from build123d import *

# Parameters (mm, degrees)
SKETCH029_W             = 70
SKETCH029_H             = 20
PAD005_DEPTH            = 12.7
SKETCH012_W             = 36
SKETCH012_H             = 17
PAD006_DEPTH            = 40
POCKET016_DEPTH         = 40
POCKET014_DEPTH         = 22.994766
SKETCH027_W             = 36
SKETCH027_H             = 30
PAD007_DEPTH            = 6
POCKET017_DEPTH         = 2
POCKET015_DEPTH         = 22
POCKET015_DEPTH_BACK    = 100
SKETCH013_R             = 9
POCKET018_DEPTH         = 40
FILLET_R                = 1
CHAMFER014_SIZE         = 2
CHAMFER013_SIZE         = 4
BODY002_ROLL_ANGLE      = -123.951696
BODY002_PITCH_ANGLE     = 0.828143
BODY002_PLACEMENT_ANGLE = 179.441913


with BuildPart() as part:
    # Sketch029 → Pad005 (new body)
    with BuildSketch(Plane.XY):
        with Locations((-8, 8)):
            Rectangle(SKETCH029_W, SKETCH029_H)
    extrude(amount=PAD005_DEPTH)

    # Sketch012 (on Face6 of Pad005) → Pad006 (join)
    with BuildSketch(Plane.XY.offset(12.7)):
        with Locations((-8, 9.5)):
            Rectangle(SKETCH012_W, SKETCH012_H)
    extrude(amount=PAD006_DEPTH)

    # Sketch028 → Pocket016 (cut)
    with BuildSketch(Plane.XY.offset(52.7)):
        with BuildLine():
            ThreePointArc((-3, 5), (-8, 10), (-13, 5))
            Line((-13, -7.39), (-13, 5))
            Line((-3, -7.39), (-13, -7.39))
            Line((-3, 5), (-3, -7.39))
        make_face()
    extrude(amount=-POCKET016_DEPTH, mode=Mode.SUBTRACT)

    # Sketch025 → Pocket014 (cut, through all)
    with BuildSketch(Plane(origin=(0, 20.993766, 0), x_dir=(-1, 0, 0), z_dir=(0, 1, 0))):
        with BuildLine():
            ThreePointArc((-16.5, 8.95), (-19.1, 6.35), (-16.5, 3.75))
            Line((-16.5, 3.75), (-14.5, 3.75))
            ThreePointArc((-14.5, 3.75), (-11.9, 6.35), (-14.5, 8.95))
            Line((-16.5, 8.95), (-14.5, 8.95))
        make_face()
        with BuildLine():
            ThreePointArc((30.5, 8.95), (27.9, 6.35), (30.5, 3.75))
            Line((30.5, 3.75), (32.5, 3.75))
            ThreePointArc((32.5, 3.75), (35.1, 6.35), (32.5, 8.95))
            Line((30.5, 8.95), (32.5, 8.95))
        make_face()
    extrude(amount=-POCKET014_DEPTH, mode=Mode.SUBTRACT)

    # Sketch027 → Pad007 (join)
    with BuildSketch(Plane.XY.offset(52.7)):
        with Locations((-8, 3)):
            Rectangle(SKETCH027_W, SKETCH027_H)
        with BuildLine():
            ThreePointArc((-19.25, -7), (-21, -5.25), (-22.75, -7))
            Line((-22.75, -7), (-22.75, -9))
            ThreePointArc((-22.75, -9), (-21, -10.75), (-19.25, -9))
            Line((-19.25, -7), (-19.25, -9))
        make_face(mode=Mode.SUBTRACT)
        with BuildLine():
            ThreePointArc((6.75, -7), (5, -5.25), (3.25, -7))
            Line((3.25, -7), (3.25, -9))
            ThreePointArc((3.25, -9), (5, -10.75), (6.75, -9))
            Line((6.75, -7), (6.75, -9))
        make_face(mode=Mode.SUBTRACT)
    extrude(amount=PAD007_DEPTH)

    # Sketch026 → Pocket017 (cut)
    with BuildSketch(Plane.XY.offset(56.7)):
        Polygon((5.856406, 5), (-1.071797, 17), (-14.928203, 17), (-21.856406, 5), (-14.928203, -7), (-1.071797, -7), align=None)
    extrude(amount=POCKET017_DEPTH, mode=Mode.SUBTRACT)

    # Sketch030 → Pocket015 (cut, two sides)
    with BuildSketch(Plane.XY.offset(12.7)) as pocket015_sk:
        with BuildLine():
            ThreePointArc((-3.5, 6), (-8, 10.5), (-12.5, 6))
            Line((-12.5, 6), (-12.5, 4))
            ThreePointArc((-12.5, 4), (-8, -0.5), (-3.5, 4))
            Line((-3.5, 6), (-3.5, 4))
        make_face()
    extrude(amount=-POCKET015_DEPTH, mode=Mode.SUBTRACT)
    extrude(pocket015_sk.sketch, amount=POCKET015_DEPTH_BACK, mode=Mode.SUBTRACT)

    # Sketch013 (on Face29 of Pocket015) → Pocket018 (cut)
    with BuildSketch(Plane.XY.offset(56.7)):
        with Locations((-8, 5)):
            Circle(SKETCH013_R)
    extrude(amount=-POCKET018_DEPTH, mode=Mode.SUBTRACT)

    # Fillet
    fillet_edges = [part.edges().sort_by_distance(p)[0] for p in [
        (0.062258, 1, 34.7),
        (-16.062258, 1, 34.7),
    ]]
    fillet(fillet_edges, radius=FILLET_R)

    # Chamfer014
    chamfer014_edges = [part.edges().sort_by_distance(p)[0] for p in [
        (10, -12, 55.7),
        (-26, -12, 55.7),
    ]]
    chamfer(chamfer014_edges, length=CHAMFER014_SIZE)

    # Chamfer013
    chamfer013_edges = [part.edges().sort_by_distance(p)[0] for p in [
        (-43, 18, 6.35),
        (27, 18, 6.35),
    ]]
    chamfer(chamfer013_edges, length=CHAMFER013_SIZE)


with BuildPart() as part_1:
    # Body002 roll: moved
    add(part.part.rotate(Axis((0, 0, 0), (1, 0, 0)), BODY002_ROLL_ANGLE))


with BuildPart() as part_2:
    # Body002 pitch: moved
    add(part_1.part.rotate(Axis((0, 0, 0), (0, 1, 0)), BODY002_PITCH_ANGLE))


with BuildPart() as part_3:
    # Body002 placement: moved
    add(part_2.part.moved(Location((-0.401038, -43.00558, -24.805855))).rotate(Axis((-0.401038, -43.00558, -24.805855), (0, 0, 1)), BODY002_PLACEMENT_ANGLE))


solid = part_3.part
Source: CAD feature listing. Evaluate the final solid. Frame: model axes, mm. A direction names the side the tool comes from. Round coordinates to 2 decimals unless told otherwise and drop trailing zeros. Use a Markdown table: item, result. Add a question column.
1. First-contact query: pin 1 (12 mm diameter, centred on y = -76, z = -53, fed in from +X); pin 2 (2 mm diameter, centred on x = -14.5, y = -42, fed in from +Z); pin 3 (12 mm diameter, centred on y = -52, z = -33, fed in from -X); pin 4 (5 mm diameter, centred on y = -57, z = -50.5, fed in from -X). Flat tips, straight axial feed; report the tip coordinate or a pass-through.
2. Set-up query: faces 1 (the cylindrical face through (-19.356, -43.59, -35.411)), 2 (the cylindrical face through (2.938, -51.632, -38.365)). Return all of +Z, -Z, +X, -X, +Y, -Y with unobstructed straight access to the full face (end or side cutting, diameter ignored); none if empty.
3. Line query: probe 1 along X at (y, z) = (-83.5, -67.5); probe 2 along Z at (x, y) = (4, -51); probe 3 along Z at (x, y) = (-6, -53.5). Output: solid intervals per line, ascending.
Derived:
| question | item | result |
|---|---|---|
| 1 | pin 1 | x = 25.79 |
| 1 | pin 2 | z = -24.81 |
| 1 | pin 3 | x = -27.43 |
| 1 | pin 4 | x = -10.21 |
| 2 | face 1 | none |
| 2 | face 2 | -Y |
| 3 | probe 1 | -10.18 to -1.54, 17 to 25.83 |
| 3 | probe 2 | -51.8 to -45.94, -42.84 to -40.33, -31.7 to -27.68 |
| 3 | probe 3 | -53.69 to -33.19, -31.96 to -29.58 |
